Part model, mm, in its own coordinate system. A direction names the side the tool comes from. Give positions to 0.01 mm unless a question says otherwise; leave off trailing zeros. Loops run counter-clockwise (first coordinate to the right, second up) from the corner with the lowest first, then second, coordinate; pieces in that order, holes last. Notation, with made-up numbers: M 18.5,11 L 61.5,11 A21 ccw 61.5,35 Z; hole C 16,70 d10. An arc over 180 degrees is marked long. Answer in a Markdown table with one row per item.
from build123d import *

# Parameters (mm, degrees)
SKETCH_1_W          = 200
SKETCH_1_H          = 100
EXTRUDE_1_DEPTH     = 10
SKETCH_2_R          = 2.5
SKETCH_2_R_2        = 5.5
SKETCH_2_R_3        = 1.4
SKETCH_2_R_4        = 4.1
CUT_EXTRUDE_1_DEPTH = 113.249721603
SKETCH_3_R          = 16
CUT_EXTRUDE_2_DEPTH = 7
FILLET_1_R          = 10
SKETCH_4_R          = 5.1
CUT_EXTRUDE_4_DEPTH = 5


with BuildPart() as part:
    # ｽｹｯﾁ1 → ﾎﾞｽ - 押し出し1 (new body)
    with BuildSketch(Plane(origin=(0, 0, 0), x_dir=(1, 0, 0), z_dir=(0, 1, 0))):
        Rectangle(SKETCH_1_W, SKETCH_1_H)
    extrude(amount=EXTRUDE_1_DEPTH)

    # ｽｹｯﾁ2 → ｶｯﾄ - 押し出し1 (cut, through all)
    with BuildSketch(Plane(origin=(0, 10, 0), x_dir=(1, 0, 0), z_dir=(0, 1, 0))):
        with Locations(Location((-92, 12, 0), (0, 0, 270))):
            Circle(SKETCH_2_R)
        with Locations(Location((-68, 12, 0), (0, 0, 270))):
            Circle(SKETCH_2_R)
        with Locations(Location((-92, -12, 0), (0, 0, 270))):
            Circle(SKETCH_2_R)
        with Locations(Location((-68, -12, 0), (0, 0, 270))):
            Circle(SKETCH_2_R)
        with Locations(Location((30, 0, 0), (0, 0, 270))):
            Circle(SKETCH_2_R_2)
        with Locations(Location((38, 0, 0), (0, 0, 270))):
            Circle(SKETCH_2_R_3)
        with Locations(Location((22, 0, 0), (0, 0, 270))):
            Circle(SKETCH_2_R_3)
        with Locations(Location((-80, 0, 0), (0, 0, 270))):
            Circle(SKETCH_2_R_4)
    extrude(amount=-CUT_EXTRUDE_1_DEPTH, mode=Mode.SUBTRACT)

    # ｽｹｯﾁ3 → ｶｯﾄ - 押し出し2 (cut)
    with BuildSketch(Plane.XZ):
        with Locations(Location((30, 0, 0), (0, 0, 270))):
            Circle(SKETCH_3_R)
    extrude(amount=-CUT_EXTRUDE_2_DEPTH, mode=Mode.SUBTRACT)

    # ﾌｨﾚｯﾄ1
    fillet_1_edges = [part.edges().sort_by_distance(p)[0] for p in [
        (100, 5, 50),
        (-100, 5, 50),
        (-100, 5, -50),
        (100, 5, -50),
    ]]
    fillet(fillet_1_edges, radius=FILLET_1_R)

    # ｽｹｯﾁ4 → ｶｯﾄ - 押し出し4 (cut)
    with BuildSketch(Plane.XZ):
        with Locations(Location((-85, 35, 0), (0, 0, 270))):
            Circle(SKETCH_4_R)
        with Locations(Location((-85, -35, 0), (0, 0, 270))):
            Circle(SKETCH_4_R)
        with Locations(Location((85, -35, 0), (0, 0, 270))):
            Circle(SKETCH_4_R)
        with Locations(Location((85, 35, 0), (0, 0, 270))):
            Circle(SKETCH_4_R)
    extrude(amount=-CUT_EXTRUDE_4_DEPTH, mode=Mode.SUBTRACT)


solid = part.part
(1) Saw through at B-B (x = -92). Write the cut outline in (y, z).
Recorded:
| item | result |
|---|---|
| outline | M 0,-49.8 L 10,-49.8 L 10,-14.5 L 0,-14.5 Z; M 0,-9.5 L 10,-9.5 L 10,9.5 L 0,9.5 Z; M 0,14.5 L 10,14.5 L 10,49.8 L 0,49.8 Z |
(2) Drill centre lines: line 1 along X through (y, z) = (8.1, 0); line 2 along X through (y, z) = (8, -1.5); line 3 along X through (y, z) = (4, 12). Where is each one in solid material? Low to high.
Recorded:
| item | result |
|---|---|
| line 1 | x = -100 to -84.1, -75.9 to 20.6, 23.4 to 24.5, 35.5 to 36.6, 39.4 to 100 |
| line 2 | x = -100 to -83.82, -76.18 to 24.71, 35.29 to 100 |
| line 3 | x = -100 to -94.5, -89.5 to -70.5, -65.5 to 19.42, 40.58 to 100 |
(3) Which spindle directions (+Z, -Z, +X, -X, +Y, -Y) get a long thin tool onto all of the face, cutting with end or side? Do faces 1 (the face through (88.4, 2.5, -31.2)), 2 (the face through (-67.9, 5.1, 9.5)). Say none if no direction does.
Recorded:
| item | result |
|---|---|
| face 1 | -Y |
| face 2 | +Y, -Y |
(4) Saw through at C-C (x = 32.5). Write the cut outline in (y, z), plus the area to 3 significant figures.
Recorded:
| item | result |
|---|---|
| outline | M 0,-50 L 10,-50 L 10,-4.9 L 7,-4.9 L 7,-15.8 L 0,-15.8 Z; M 0,15.8 L 7,15.8 L 7,4.9 L 10,4.9 L 10,50 L 0,50 Z |
| area | 749 mm^2 |
(5) Saw through at A-A (z = 11.5). Write the cut outline in (x, y), plus the area to 3 significant figures.
Recorded:
| item | result |
|---|---|
| outline | M -100,0 L -94.45,0 L -94.45,10 L -100,10 Z; M -89.55,0 L -70.45,0 L -70.45,10 L -89.55,10 Z; M -65.55,0 L 18.88,0 L 18.88,7 L 41.12,7 L 41.12,0 L 100,0 L 100,10 L -65.55,10 Z |
| area | 1,750 mm^2 |
(6) Pin check, flat tips, straight feed: pin 1 Ø3 at (x, z) = (-68, -12) entering from +Y; pin 2 Ø3.5 at (x, z) = (22, 0) entering from -Y; pin 3 Ø8 at (x, z) = (85, 35) entering from -Y. Stop position of each tip, or through.
Recorded:
| item | result |
|---|---|
| pin 1 | passes through |
| pin 2 | stops at y = 7 |
| pin 3 | stops at y = 5 |
(7) Saw through at D-D (x = 85). Write the cut outline in (y, z), plus the area to 3 significant figures.
Recorded:
| item | result |
|---|---|
| outline | M 0,-50 L 10,-50 L 10,50 L 0,50 L 0,40.1 L 5,40.1 L 5,29.9 L 0,29.9 L 0,-29.9 L 5,-29.9 L 5,-40.1 L 0,-40.1 Z |
| area | 898 mm^2 |
(8) Pull direction X, two halves, no side cores. Call faces 3 (the face through (100, 5, 1)), 4 (the face through (-85, 5, -35)), 5 (the face through (-1, 0, -1)): +X half, -X half, draft (parallel to the pull), parting line (faces both ways), or undercut.
Recorded:
| item | result |
|---|---|
| face 3 | +X half |
| face 4 | undercut |
| face 5 | draft |
